The listing builds one solid part. Answer for the finished solid, in the listing's coordinates (mm). Round coordinates to 2 decimals unless told otherwise and drop trailing zeros. Order: outer loops, then holes, each group sorted by start corner. A loop starts at its lowest first (then second) coordinate and runs counter-clockwise, first axis right, second up. Notation, with made-up numbers: (41.25, 72.25) -> (77.25, 72.25) arc R23 cw to (77.25, 81.25) -> close; hole circle Ø2 at (24.5, 83.5). An arc over 180 degrees is marked (long way). Return JSON: item names as keys, results as strings. Group by question number.
(1) Each of these flat-tipped pins is pushed along its axis until it touches: pin 1 (15 mm diameter, centred on y = -28, z = -261, fed in from -X); pin 2 (10 mm diameter, centred on y = -139, z = -169.5, fed in from +X); pin 3 (3 mm diameter, centred on x = 287.5, z = -339, fed in from -Y). Where does it stop, or does it pass through?
(2) The part is cut by section B-B (x = 532). Determine the outline of the cut face in (y, z), plus the area to 3 significant figures.
(3) The part is cut by section C-C (y = -505). Determine the outline of the cut face in (x, z).
(4) Consider line 1 (Y direction, x = 322, z = -254); line 2 (Z direction, x = 311, y = -63); line 3 (Y direction, x = 320, z = -110). Determine where each line is inside the solid, lowest interval first. Write a range as [from, to].
(5) The part is cut by section A-A (z = -324.5). Determine the outline of the cut face in (x, y).
from build123d import *

# Parameters (mm, degrees)
SKETCH1_W           = 381
SKETCH1_H           = 508
BOSS_EXTRUDE1_DEPTH = 12.7
SKETCH3_R           = 6.35
BOSS_EXTRUDE2_DEPTH = 12.7
BOSS_EXTRUDE4_DEPTH = 508


with BuildPart() as part:
    # Sketch1 → Boss-Extrude1 (new body)
    with BuildSketch(Plane(origin=(0, 0, 0), x_dir=(1, 0, 0), z_dir=(0, 1, 0))):
        with Locations((317.5, 254)):
            Rectangle(SKETCH1_W, SKETCH1_H)
    extrude(amount=BOSS_EXTRUDE1_DEPTH)

    # Sketch3 → Boss-Extrude2 (add, symmetric)
    with BuildSketch(Plane(origin=(317.5, 0, 0), x_dir=(0, 0, -1), z_dir=(1, 0, 0))):
        with BuildLine():
            Line((228.6, 0), (228.6, -63.5))
            ThreePointArc((228.6, -63.5), (254, -88.9), (279.4, -63.5))
            Line((279.4, -63.5), (279.4, 0))
            Line((279.4, 0), (228.6, 0))
        make_face()
        with Locations((254, -63.5)):
            Circle(SKETCH3_R, mode=Mode.SUBTRACT)
    extrude(amount=BOSS_EXTRUDE2_DEPTH, both=True)

    # Sketch6 → Boss-Extrude4 (add)
    with BuildSketch(Plane.XY):
        Polygon((520.7, 12.7), (608.913274255, -487.58233853), (834.18077195, -645.31633853), (819.241419295, -645.31633853), (593.9739216, -487.58233853), (508, 0), (508, 12.7), align=None)
    extrude(amount=-BOSS_EXTRUDE4_DEPTH)


solid = part.part
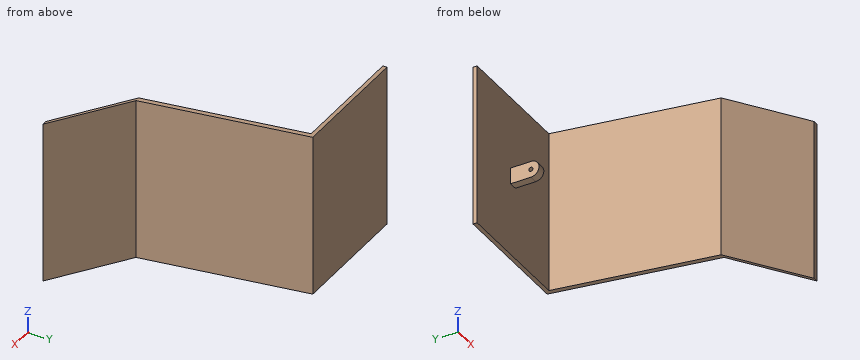
Answer below:
{
 "1": {"pin 1": "stops at x = 304.8", "pin 2": "stops at x = 548.33", "pin 3": "stops at y = 0"},
 "2": {"outline": "(-136.11, -508) -> (-51.39, -508) -> (-51.39, 0) -> (-136.11, 0) -> close", "area": "43,000 mm²"},
 "3": {"outline": "(618.85, -508) -> (633.79, -508) -> (633.79, 0) -> (618.85, 0) -> close"},
 "4": {"line 1": "y = [-88.9, -69.85], [-57.15, 12.7]", "line 2": "z = [-279.4, -260.33], [-247.67, -228.6]", "line 3": "y = [0, 12.7]"},
 "5": {"outline": "(127, 0) -> (508, 0) -> (593.97, -487.58) -> (819.24, -645.32) -> (834.18, -645.32) -> (608.91, -487.58) -> (520.7, 12.7) -> (127, 12.7) -> close"}
}
